from build123d import *

# Parameters (mm, degrees)
CYLINDER014_R     = 9.8
CYLINDER014_DEPTH = 10
CYLINDER013_R     = 10.3
CYLINDER013_DEPTH = 10
CYLINDER012_R     = 11.05
CYLINDER012_DEPTH = 5


with BuildPart() as redtmp04:
    # Cylinder014 → Cylinder014 (new body)
    with BuildSketch(Plane.XY):
        Circle(CYLINDER014_R)
    extrude(amount=CYLINDER014_DEPTH)


with BuildPart() as redtmp02:
    # Cylinder013 → Cylinder013 (new body)
    with BuildSketch(Plane.XY.offset(0.5)):
        Circle(CYLINDER013_R)
    extrude(amount=CYLINDER013_DEPTH)


with BuildPart() as redbase:
    # Cylinder012 → Cylinder012 (new body)
    with BuildSketch(Plane.XY):
        Circle(CYLINDER012_R)
    extrude(amount=CYLINDER012_DEPTH)

    # Cut008: cut RedTmp02
    add(redtmp02.part, mode=Mode.SUBTRACT)

    # Cut009: cut RedTmp04
    add(redtmp04.part, mode=Mode.SUBTRACT)


with BuildPart() as redbase_1:
    # Cut009 placement: moved
    add(redbase.part.moved(Location((10, 40, 0))))


solid = redbase_1.part
Work out the finished part from the listing and answer in its coordinate system (mm). A direction names the side the tool comes from. Round coordinates to 2 decimals unless told otherwise and drop trailing zeros. Write each loop counter-clockwise with the first axis right and the second up, starting at its lowest first coordinate (ties: lowest second). Pieces come first, ordered by that corner, then holes. Notation, with made-up numbers: (42, 89.25) -> (90, 89.25) arc R14 cw to (90, 99.25) -> close; hole circle Ø7 at (70, 49.5). An arc over 180 degrees is marked (long way). Write each question's results on one line, items separated by ' | '.
Item 1: The mould has two halves that part along Y. Classify faces 1 (the face through (20, 40, 0.5)), 2 (the face through (15.94, 49.32, 2.46)), 3 (the face through (9, 30, 0)): +Y half, -Y half, draft (parallel to the pull), parting line (faces both ways), or undercut.
Result set:
face 1: undercut | face 2: parting line | face 3: draft
Item 2: Flat-ended cylindrical pins translate along their axes: P1, Ø1.5, axis at y = 48, z = 4, coming from the -X side; P2, Ø3, axis at y = 42.5, z = 2.5, coming from the +X side; P3, Ø2, axis at x = 2.5, y = 41, coming from the +Z side; P4, Ø3, axis at x = 16, z = 1, coming from the +Y side. Find the tip coordinate at first contact, or state that the pin passes through.
Result set:
P1: x = 1.66 | P2: x = 21 | P3: through | P4: y = 50.09
Item 3: Find the intervals of material crossed by line 1 along X through (y, z) = (39.75, 2.8); line 2 along Y through (x, z) = (10, 2.6); line 3 along Y through (x, z) = (10, 0.15), in increasing order. Write a range as [from, to].
Result set:
line 1: [-1.05, -0.3], [20.3, 21.05] | line 2: [28.95, 29.7], [50.3, 51.05] | line 3: [28.95, 30.2], [49.8, 51.05]
Item 4: A cutting plane is placed at B-B, the plane x = 10. Determine the outline of the cut face in (y, z).
Result set:
outline: (28.95, 0) -> (30.2, 0) -> (30.2, 0.5) -> (29.7, 0.5) -> (29.7, 5) -> (28.95, 5) -> close; (49.8, 0) -> (51.05, 0) -> (51.05, 5) -> (50.3, 5) -> (50.3, 0.5) -> (49.8, 0.5) -> close
Item 5: Which of the six approach directions +Z, -Z, +X, -X, +Y, -Y give full straight-line access (tool end or side, diameter ignored) to faces 4 (the face through (7.876, 30.433, 0.246)), 5 (the face through (7.767, 29.945, 2.718))?
Result set:
face 4: +Z, -Z | face 5: +Z
Item 6: A cutting plane is placed at C-C, the plane z = 3.55. Determine the outline of the cut face in (x, y).
Result set:
outline: circle Ø22.1 at (10, 40); hole circle Ø20.6 at (10, 40)
Item 7: A cutting plane is placed at A-A, the plane y = 40. Determine the outline of the cut face in (x, z), plus the area to 3 significant figures.
Result set:
outline: (-1.05, 0) -> (0.2, 0) -> (0.2, 0.5) -> (-0.3, 0.5) -> (-0.3, 5) -> (-1.05, 5) -> close; (19.8, 0) -> (21.05, 0) -> (21.05, 5) -> (20.3, 5) -> (20.3, 0.5) -> (19.8, 0.5) -> close | area: 8.00 mm^2
